Here's how the part is built. I have some questions about the finished solid (model axes, mm). Face numbers are marked on the shaded views. A direction names the side the tool comes from. Give positions to 0.01 mm unless a question says otherwise; leave off trailing zeros. Loops run counter-clockwise (first coordinate to the right, second up) from the corner with the lowest first, then second, coordinate; pieces in that order, holes last. Notation, with made-up numbers: (62.5, 77) - (111.5, 77) arc R19 cw to (111.5, 104) - close; hole circle Ø7 at (-8, 24). An arc over 180 degrees is marked (long way). Return JSON: item names as keys, results as strings. Group by question number.
(1) On a 3-axis mill with a long thin cutter (end or side, diameter ignored), from which of +Z, -Z, +X, -X, +Y, -Y can I reach the whole of each face in a straight line? I mean the marked faces 1 and 2. Say none if no direction works.
(2) For P1, Ø3, axis at x = -1.5, z = 1, coming from the -Y side; P2, Ø1.8, axis at y = -11.5, z = 4, coming from the -X side; P3, Ø1.8, axis at y = -13.5, z = 1.5, coming from the +X side, each with a flat end and sliding along its axis, tell me the tip position at first contact or that it passes through.
(3) If we section it at C-C (y = 4): Please give me the cut outline in (x, z).
(4) If we section it at A-A (x = -2): Please give me the cut outline in (y, z).
(5) If we section it at B-B (y = -17.5): Please give me the cut outline in (x, z).
(6) If we mould it in two halves opening along X, with no side actions, what happens to the marked faces 3, 4 and 5? For each: released by +X, released by -X, zero draft, split by the parting line, or undercut.
(7) If we section it at D-D (z = 3.7): State how many separate pieces and enclosed holes the cut face has, then the cut area to 3 significant figures.
(8) I need wall thicknesses on probe 1 along Y at (x, z) = (0, 4.2); probe 2 along Y at (x, z) = (6, 4.2); probe 3 along X at (y, z) = (-17.5, 5.4). Which ranges of each line are inside material? Lowest first, please. Write a range as [from, to].
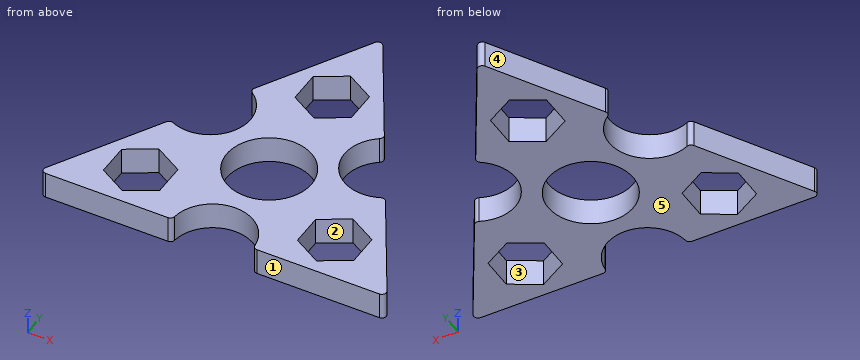
```python
from build123d import *

# Parameters (mm, degrees)
F0_R     = 9.45
F1_DEPTH = 6
F2_R     = 1
F3_R     = 1


with BuildPart() as f1:
    # F0 (on Top) → F1 (new body)
    with BuildSketch(Plane.XY):
        with BuildLine():
            Line((14.9855715851, 19.0442286341), (0, 45))
            Line((0, 45), (-14.9855715851, 19.0442286341))
            ThreePointArc((-14.9855715851, 19.0442286341), (-11.6913429511, 6.75), (-23.9855715851, 3.4557713659))
            Line((-23.9855715851, 3.4557713659), (-38.9711431703, -22.5))
            Line((-38.9711431703, -22.5), (-9, -22.5))
            ThreePointArc((-9, -22.5), (0, -13.5), (9, -22.5))
            Line((9, -22.5), (38.9711431703, -22.5))
            Line((38.9711431703, -22.5), (23.9855715851, 3.4557713659))
            ThreePointArc((23.9855715851, 3.4557713659), (11.6913429511, 6.75), (14.9855715851, 19.0442286341))
        make_face()
        Polygon((-15.3719509172, -16.125), (-21.6506350946, -19.75), (-27.929319272, -16.125), (-27.929319272, -8.875), (-21.6506350946, -5.25), (-15.3719509172, -8.875), align=None, mode=Mode.SUBTRACT)
        Polygon((21.6506350946, -5.25), (27.929319272, -8.875), (27.929319272, -16.125), (21.6506350946, -19.75), (15.3719509172, -16.125), (15.3719509172, -8.875), align=None, mode=Mode.SUBTRACT)
        Circle(F0_R, mode=Mode.SUBTRACT)
        Polygon((-6.2786841774, 28.625), (0, 32.25), (6.2786841774, 28.625), (6.2786841774, 21.375), (0, 17.75), (-6.2786841774, 21.375), align=None, mode=Mode.SUBTRACT)
    extrude(amount=F1_DEPTH)

    # F2
    f2_edges = [f1.edges().sort_by_distance(p)[0] for p in [
        (14.985572, 19.044229, 3),
        (-23.985572, 3.455771, 3),
        (9, -22.5, 3),
    ]]
    fillet(f2_edges, radius=F2_R)

    # F3
    f3_edges = [f1.edges().sort_by_distance(p)[0] for p in [
        (0, 45, 3),
        (38.971143, -22.5, 3),
        (-38.971143, -22.5, 3),
        (-14.985572, 19.044229, 3),
        (23.985572, 3.455771, 3),
        (-9, -22.5, 3),
    ]]
    fillet(f3_edges, radius=F3_R)


solid = f1.part
```
Values:
{
 "1": {"face 1": "+Z, -Z, +X, -X, -Y", "face 2": "+Z, -Z"},
 "2": {"P1": "y = -14.01", "P2": "x = -33.14", "P3": "x = 34.29"},
 "3": {"outline": "(-14.15, 0) - (-8.56, 0) - (-8.56, 6) - (-14.15, 6) - close; (8.56, 0) - (14.15, 0) - (14.15, 6) - (8.56, 6) - close"},
 "4": {"outline": "(-13.73, 0) - (-9.24, 0) - (-9.24, 6) - (-13.73, 6) - close; (9.24, 0) - (18.9, 0) - (18.9, 6) - (9.24, 6) - close; (31.1, 0) - (41.54, 0) - (41.54, 6) - (31.1, 6) - close"},
 "5": {"outline": "(-36.08, 0) - (-25.55, 0) - (-25.55, 6) - (-36.08, 6) - close; (-17.75, 0) - (-7.48, 0) - (-7.48, 6) - (-17.75, 6) - close; (7.48, 0) - (17.75, 0) - (17.75, 6) - (7.48, 6) - close; (25.55, 0) - (36.08, 0) - (36.08, 6) - (25.55, 6) - close"},
 "6": {"face 3": "undercut", "face 4": "released by -X", "face 5": "zero draft"},
 "7": {"separate pieces": "1", "enclosed holes": "4", "area": "1,560 mm2"},
 "8": {"probe 1": "[-13.5, -9.45], [9.45, 17.75], [32.25, 44]", "probe 2": "[-15.79, -7.3], [7.3, 21.21], [28.79, 34.61]", "probe 3": "[-36.08, -25.55], [-17.75, -7.48], [7.48, 17.75], [25.55, 36.08]"}
}
